Geometry check sheet. Reference: the model listing, model coordinates, mm. Coordinates: 2 decimals unless noted, no trailing zeros. Loops run counter-clockwise (first coordinate to the right, second up) from the corner with the lowest first, then second, coordinate; pieces in that order, holes last.
from build123d import *

# Parameters (mm, degrees)
F0_R     = 2.54
F1_DEPTH = 1.27
F3_DEPTH = 25.4


with BuildPart() as f1:
    # F0 (on Top) → F1 (new body)
    with BuildSketch(Plane.XY):
        with BuildLine():
            ThreePointArc((-94.472359, -11.035805), (-97.203597, -12.591866), (-97.257687, -15.734805))
            ThreePointArc((-97.257687, -15.734805), (-36.546229, -50.36885), (21.726042, -11.771693))
            ThreePointArc((21.726042, -11.771693), (22.194683, -11.235473), (22.878268, -11.035805))
            Line((22.878268, -11.035805), (25.526176, -11.035805))
            add(Edge.make_bspline(
                [(26.63919, -11.035805), (26.515522, -11.035805), (26.268185, -11.035805), (25.897181, -11.035805), (25.649844, -11.035805), (25.526176, -11.035805)],
                knots=[0, 0, 0, 0, 0.371005, 0.742009, 1.113014, 1.113014, 1.113014, 1.113014], degree=3))
            Line((26.63919, -11.035805), (26.636754, -3.015521))
            Line((26.636754, -3.015521), (15.20919, -3.015521))
            Line((15.20919, -3.015521), (15.206754, -3.015521))
            Line((15.206754, -3.015521), (13.68519, -3.015521))
            Line((13.68519, -3.015521), (13.68519, -11.035805))
            Line((13.68519, -11.035805), (-19.2116, -11.035805))
            Line((-19.2116, -11.035805), (-19.776128, -7.834206))
            ThreePointArc((-19.776128, -7.834206), (-23.528246, -4.685805), (-27.280363, -7.834206))
            Line((-27.280363, -7.834206), (-27.844892, -11.035805))
            Line((-27.844892, -11.035805), (-33.688246, -11.035805))
            Line((-33.688246, -11.035805), (-49.6916, -11.035805))
            Line((-49.6916, -11.035805), (-50.256128, -7.834206))
            ThreePointArc((-50.256128, -7.834206), (-54.008246, -4.685805), (-57.760363, -7.834206))
            Line((-57.760363, -7.834206), (-58.324892, -11.035805))
            Line((-58.324892, -11.035805), (-64.168246, -11.035805))
            Line((-64.168246, -11.035805), (-94.472359, -11.035805))
        make_face()
        with Locations((-54.008246, -8.495805)):
            Circle(F0_R, mode=Mode.SUBTRACT)
        with Locations((-23.528246, -8.495805)):
            Circle(F0_R, mode=Mode.SUBTRACT)
    extrude(amount=F1_DEPTH)

    # F2 (on face) → F3 (cut)
    with BuildSketch(Plane.XY.offset(1.27)):
        with BuildLine():
            ThreePointArc((-81.137359, -12.305805), (-81.772359, -11.670805), (-82.407359, -12.305805))
            Line((-82.407359, -12.305805), (-82.407359, -31.355805))
            ThreePointArc((-82.407359, -31.355805), (-81.772359, -31.990805), (-81.137359, -31.355805))
            Line((-81.137359, -31.355805), (-81.137359, -12.305805))
        make_face()
        with BuildLine():
            ThreePointArc((-71.462298, -12.305805), (-72.097298, -11.670805), (-72.732298, -12.305805))
            Line((-72.732298, -12.305805), (-72.732298, -31.355805))
            ThreePointArc((-72.732298, -31.355805), (-72.097298, -31.990805), (-71.462298, -31.355805))
            Line((-71.462298, -31.355805), (-71.462298, -12.305805))
        make_face()
        with BuildLine():
            ThreePointArc((-61.787237, -12.305805), (-62.422237, -11.670805), (-63.057237, -12.305805))
            Line((-63.057237, -12.305805), (-63.057237, -31.355805))
            ThreePointArc((-63.057237, -31.355805), (-62.422237, -31.990805), (-61.787237, -31.355805))
            Line((-61.787237, -31.355805), (-61.787237, -12.305805))
        make_face()
        with BuildLine():
            ThreePointArc((-52.112176, -12.305805), (-52.747176, -11.670805), (-53.382176, -12.305805))
            Line((-53.382176, -12.305805), (-53.382176, -31.355805))
            ThreePointArc((-53.382176, -31.355805), (-52.747176, -31.990805), (-52.112176, -31.355805))
            Line((-52.112176, -31.355805), (-52.112176, -12.305805))
        make_face()
        with BuildLine():
            ThreePointArc((-42.437115, -12.305805), (-43.072115, -11.670805), (-43.707115, -12.305805))
            Line((-43.707115, -12.305805), (-43.707115, -31.355805))
            ThreePointArc((-43.707115, -31.355805), (-43.072115, -31.990805), (-42.437115, -31.355805))
            Line((-42.437115, -31.355805), (-42.437115, -12.305805))
        make_face()
        with BuildLine():
            ThreePointArc((-32.762054, -12.305805), (-33.397054, -11.670805), (-34.032054, -12.305805))
            Line((-34.032054, -12.305805), (-34.032054, -31.355805))
            ThreePointArc((-34.032054, -31.355805), (-33.397054, -31.990805), (-32.762054, -31.355805))
            Line((-32.762054, -31.355805), (-32.762054, -12.305805))
        make_face()
        with BuildLine():
            ThreePointArc((-23.086993, -12.305805), (-23.721993, -11.670805), (-24.356993, -12.305805))
            Line((-24.356993, -12.305805), (-24.356993, -31.355805))
            ThreePointArc((-24.356993, -31.355805), (-23.721993, -31.990805), (-23.086993, -31.355805))
            Line((-23.086993, -31.355805), (-23.086993, -12.305805))
        make_face()
        with BuildLine():
            ThreePointArc((-13.411932, -12.305805), (-14.046932, -11.670805), (-14.681932, -12.305805))
            Line((-14.681932, -12.305805), (-14.681932, -31.355805))
            ThreePointArc((-14.681932, -31.355805), (-14.046932, -31.990805), (-13.411932, -31.355805))
            Line((-13.411932, -31.355805), (-13.411932, -12.305805))
        make_face()
        with BuildLine():
            ThreePointArc((-3.736871, -12.305805), (-4.371871, -11.670805), (-5.006871, -12.305805))
            Line((-5.006871, -12.305805), (-5.006871, -31.355805))
            ThreePointArc((-5.006871, -31.355805), (-4.371871, -31.990805), (-3.736871, -31.355805))
            Line((-3.736871, -31.355805), (-3.736871, -12.305805))
        make_face()
        with BuildLine():
            ThreePointArc((5.93819, -12.305805), (5.30319, -11.670805), (4.66819, -12.305805))
            Line((4.66819, -12.305805), (4.66819, -31.355805))
            ThreePointArc((4.66819, -31.355805), (5.30319, -31.990805), (5.93819, -31.355805))
            Line((5.93819, -31.355805), (5.93819, -12.305805))
        make_face()
    extrude(amount=-F3_DEPTH, mode=Mode.SUBTRACT)


solid = f1.part
(1) Draft check along Y on faces 1 (the cylindrical face through (-97.18, -12.55, 0.63)), 2 (the cylindrical face through (-56.546, -8.384, 0.626)), 3 (the flat face through (-36, -26, 0)). Enter one of: +Y half, -Y half, draft (parallel to the pull), parting line (faces both ways), or undercut.
Findings:
face 1: parting line
face 2: undercut
face 3: draft
(2) Sectioned sample at B-B on x = -88. Record the cut outline in (y, z).
Findings:
outline: (-28.69, 0) - (-11.04, 0) - (-11.04, 1.27) - (-28.69, 1.27) - close
(3) Sectioned sample at A-A on y = -20.5. State how many separate pieces and enclosed holes the cut face has, and give its area (3 significant figures).
Findings:
separate pieces: 11
enclosed holes: 0
area: 125 mm2
(4) Gauge pin test, flat end, axial feed: pin 1 Ø0.6 at (y, z) = (-23.5, 0.5) entering from -X. Record the tip position at first contact, or that the pin passes through.
Findings:
pin 1: stops at x = -92.5
(5) Scan lines: L1, parallel to X at y = -39.5, z = 0.7; L2, parallel to Y at x = -47, z = 1.2; L3, parallel to X at y = -40.5, z = 0.5. Record each from-to range of solid material in increasing order.
Findings:
L1: x = -75.31 to -2.22
L2: y = -49.9 to -11.04
L3: x = -73.73 to -3.8
